Build history of the part. All positions in model axes, mm. A direction names the side the tool comes from. Coordinates: 2 decimals unless noted, no trailing zeros. Order: outer loops, then holes, each group sorted by start corner. A loop starts at its lowest first (then second) coordinate and runs counter-clockwise, first axis right, second up. Notation, with made-up numbers: (89.5, 77) - (97.5, 77) arc R20 ccw to (97.5, 116) - close; hole circle Ø11 at (-32, -39). An arc over 180 degrees is marked (long way). Write each question's results on one line, items separated by ' | '.
from build123d import *

# Parameters (mm, degrees)
F1_ANGLE = 180
F3_DEPTH = 35


with BuildPart() as f1:
    # F0 (on Front) → F1 (revolve)
    with BuildSketch(Plane.XZ):
        with BuildLine():
            ThreePointArc((0, 25), (17.67767, 17.67767), (25, 0))
            Line((25, 0), (25.5, 0))
            ThreePointArc((25.5, 0), (18.031223, 18.031223), (0, 25.5))
            Line((0, 25.5), (0, 25))
        make_face()
        with BuildLine():
            Line((25.5, 0), (25, 0))
            ThreePointArc((25, 0), (24.622145, -4.330127), (23.5, -8.529361))
            Line((23.5, -8.529361), (23.5, -17))
            Line((23.5, -17), (25.5, -17))
            Line((25.5, -17), (25.5, 0))
        make_face()
    revolve(axis=Axis((0, 0, 9.860388), (0, 0, -1)), revolution_arc=F1_ANGLE)

    # F2 (on face) → F3 (join)
    with BuildSketch(Plane(origin=(0, 0, 0), x_dir=(-1, 0, 0), z_dir=(0, 1, 0))):
        with BuildLine():
            ThreePointArc((25.5, 0), (0, 25.5), (-25.5, 0))
            Line((-25.5, 0), (-25.5, -17))
            Line((-25.5, -17), (-23.5, -17))
            Line((-23.5, -17), (-23.5, -8.529361))
            ThreePointArc((-23.5, -8.529361), (0, 25), (23.5, -8.529361))
            Line((23.5, -8.529361), (23.5, -17))
            Line((23.5, -17), (25.5, -17))
            Line((25.5, -17), (25.5, 0))
        make_face()
    extrude(amount=F3_DEPTH)


solid = f1.part
1. Drop flat-ended pins along their axis: pin 1 Ø3 at (x, z) = (-20, 3.5) entering from -Y; pin 2 Ø8 at (x, y) = (9, -13) entering from -Z; pin 3 Ø4 at (y, z) = (-12.5, 19) entering from +X. Give the stop position or say it passes through.
Solved:
pin 1: stops at y = -17.22 | pin 2: stops at z = 15.25 | pin 3: stops at x = 14.83
2. Band-saw the part on B-B on z = -12.5. Give the cut face in (x, y).
Solved:
outline: (-25.5, 0) arc R25.5 ccw to (25.5, 0) - (25.5, 35) - (23.5, 35) - (23.5, 0) arc R23.5 cw to (-23.5, 0) - (-23.5, 35) - (-25.5, 35) - close
3. Two-plate mould, pull along X, no slides. Class faces 3 (the face through (23.5, 17, -13)), 4 (the face through (15.2, 35, 20.1)), 5 (the face through (-0.561, 17.255, 25.494)), 6 (the face through (0.67, 17.26, 24.99)): +X half, -X half, draft (parallel to the pull), parting line (faces both ways), or undercut.
Solved:
face 3: undercut | face 4: draft | face 5: parting line | face 6: undercut
4. Tool access for faces 1 (the face through (-25.5, 17, -9)), 2 (the face through (-23.5, 17, -13)): list every direction of +Z, -Z, +X, -X, +Y, -Y with a clear straight run to the whole face (end or side of a thin tool).
Solved:
face 1: +Z, -Z, -X, +Y, -Y | face 2: -Z, +Y
5. Probe line 1 (Z direction, x = 0, y = 15); line 2 (X direction, y = -3.5, z = 22); line 3 (X direction, y = 1, z = 15.5). List the from-to ranges inside material, lowest first.
Solved:
line 1: z = 25 to 25.5 | line 2: x = -12.41 to -11.35, 11.35 to 12.41 | line 3: x = -20.25 to -19.62, 19.62 to 20.25
6. Band-saw the part on A-A on y = 26. Give the cut face in (x, z), then the cut area to 3 significant figures.
Solved:
outline: (-25.5, -17) - (-23.5, -17) - (-23.5, -8.53) arc R25 cw (long way) to (23.5, -8.53) - (23.5, -17) - (25.5, -17) - (25.5, 0) arc R25.5 ccw to (-25.5, 0) - close | area: 90.5 mm2
